Solid Edge part; units mm, degrees
sketch "Sketch1" plane through (0, 0, 0) normal (0, 0, 1) x (1, 0, 0)
  circle A0 centre (0, 0) radius 60
extrude "Protrusion1" add sketch "Sketch1" against normal blind 275
sketch "Sketch2" plane through (0, 0, 0) normal (0, 0, 1) x (1, 0, 0)
  circle A0 centre (0, 0) radius 59
extrude "Cutout1" cut sketch "Sketch2" against normal up to next
sketch "Sketch3" plane through (0, -98.8326, 0) normal (0, -1, 0) x (1, 0, 0)
  line L0 (-22.5, -250) -> (22.5, -250)
  line L1 (22.5, -250) -> (22.5, -25)
  line L2 (22.5, -25) -> (-22.5, -25)
  line L3 (-22.5, -25) -> (-22.5, -250)
  dimension "D1" = 22.5
extrude "Cutout2" cut sketch "Sketch3" against normal blind 261.0003
sketch "Sketch4" plane through (116.4196, 0, 0) normal (1, 0, 0) x (0, 1, 0)
  line L0 (-22.5, -250) -> (22.5, -250)
  line L1 (22.5, -250) -> (22.5, -25)
  line L2 (22.5, -25) -> (-22.5, -25)
  line L3 (-22.5, -25) -> (-22.5, -250)
  dimension "D1" = 22.5
extrude "ExtrudedCutout_5" cut sketch "Sketch4" against normal blind 221.6217
properties material "Acrylic Plastic (extra strong)"
Input: part model. Units: mm. Frame: model coordinates. Give positions to 0.01 mm unless a question says otherwise; leave off trailing zeros. Order: outer loops, then holes, each group sorted by start corner. A loop starts at its lowest first (then second) coordinate and runs counter-clockwise, first axis right, second up. Notation, with made-up numbers: (14.5, 77.25) - (67.5, 77.25) arc R33 ccw to (67.5, 108.25) - close; hole circle Ø3 at (44, -29.5). An arc over 180 degrees is marked (long way). Answer as a JSON object with one key per item and string values. Group by question number.
Q1. Mould query, pull axis X, two halves, no side actions, for faces 1 (the face through (27.225, -52.343, -135.575)), 2 (the face through (59.3, 0.1, -25)), 3 (the face through (27.69, -53.23, -135.57)). Classes: pulls with the +X half, pulls with the -X half, needs draft (parallel to the pull), parting line crosses it, or undercut.
Q2. Cut plane C-C, the plane y = 51. Output: boundary loops of the cut face in (x, z).
Q3. First-contact query: pin 1 Ø2 at (x, z) = (23, -65) entering from -Y; pin 2 Ø0.5 at (x, z) = (-55, -102.5) entering from +Y; pin 3 Ø0.9 at (x, z) = (55.5, -171) entering from +Y. Flat tips, straight axial feed; report the tip coordinate or a pass-through.
Q4. Cut plane A-A, the plane y = 0. Output: boundary loops of the cut face in (x, z), then the cut area to 3 significant figures.
Q5. Cut plane D-D, the plane x = 28. Output: boundary loops of the cut face in (y, z).
Q6. Line query: probe 1 along Y at (x, z) = (40.5, -255); probe 2 along Y at (x, z) = (41.5, -110); probe 3 along X at (y, z) = (23.5, -252.5). Output: solid intervals per line, ascending.
Results:
{
 "1": {"face 1": "undercut", "face 2": "needs draft", "face 3": "parting line crosses it"},
 "2": {"outline": "(-31.61, -275) - (-29.66, -275) - (-29.66, 0) - (-31.61, 0) - close; (29.66, -275) - (31.61, -275) - (31.61, 0) - (29.66, 0) - close"},
 "3": {"pin 1": "y = -55.62", "pin 2": "y = 24.54", "pin 3": "y = 23.86"},
 "4": {"outline": "(-60, -275) - (-59, -275) - (-59, -250) - (-60, -250) - close; (-60, -25) - (-59, -25) - (-59, 0) - (-60, 0) - close; (59, -275) - (60, -275) - (60, -250) - (59, -250) - close; (59, -25) - (60, -25) - (60, 0) - (59, 0) - close", "area": "100 mm^2"},
 "5": {"outline": "(-53.07, -275) - (-51.93, -275) - (-51.93, 0) - (-53.07, 0) - close; (51.93, -275) - (53.07, -275) - (53.07, 0) - (51.93, 0) - close"},
 "6": {"probe 1": "-44.27 to -42.9, 42.9 to 44.27", "probe 2": "-43.33 to -41.94, 41.94 to 43.33", "probe 3": "-55.21 to -54.12, 54.12 to 55.21"}
}
